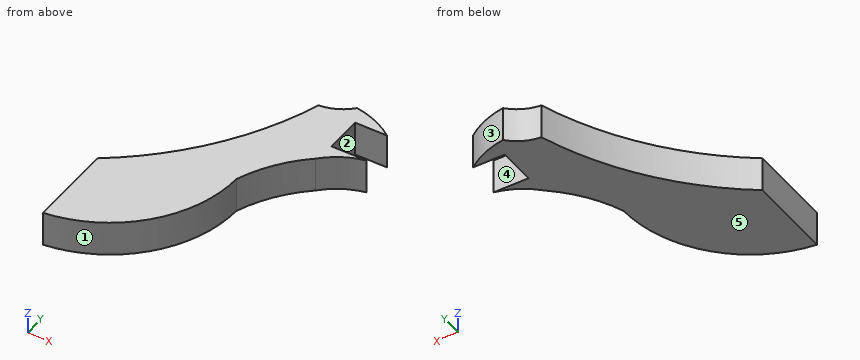
from build123d import *

# Parameters (mm, degrees)
BOSS_EXTRUDE1_DEPTH = 1.524


with BuildPart() as part:
    # Sketch1 → Boss-Extrude1 (new body)
    with BuildSketch(Plane.XY):
        with BuildLine():
            Line((110.824360774, -1.524), (109.29292347, -1.524))
            Line((109.29292347, -1.524), (109.29292347, 0.099254425))
            Line((109.29292347, 0.099254425), (110.685720546, 0.099254425))
            ThreePointArc((110.685720546, 0.099254425), (109.844126395, 0.589914025), (108.904790048, 0.848128638))
            ThreePointArc((108.904790048, 0.848128638), (108.321557599, 0.411980775), (107.618800979, 0.220883469))
            ThreePointArc((107.618800979, 0.220883469), (105.564728066, -3.682348009), (102.379001913, -6.732852948))
            Line((102.379001913, -6.732852948), (102.379001913, -10.469177864))
            ThreePointArc((102.379001913, -10.469177864), (105.901664911, -8.680555585), (107.348345234, -5.004220414))
            ThreePointArc((107.348345234, -5.004220414), (108.094332128, -3.601037602), (109.178159994, -2.438826088))
            ThreePointArc((109.178159994, -2.438826088), (109.930755444, -1.854541621), (110.824360774, -1.524))
        make_face()
    extrude(amount=BOSS_EXTRUDE1_DEPTH)


solid = part.part
For this review, take the finished solid that the model builds, in its own axes (mm). Face numbers are marked on the shaded views. A direction names the side the tool comes from. Round coordinates to 2 decimals unless told otherwise and drop trailing zeros. Loops run counter-clockwise (first coordinate to the right, second up) from the corner with the lowest first, then second, coordinate; pieces in that order, holes last. Notation, with made-up numbers: (89.25, 46) - (121.25, 46) arc R24 ccw to (121.25, 79) - close; hole circle Ø4 at (73.5, 68.5). An arc over 180 degrees is marked (long way). One line per question, with ' | ' between items.
Q1. For line 1 along X through (y, z) = (-7.25, 1.1); line 2 along Y through (x, z) = (103, 0.7); line 3 along Y through (x, z) = (106.25, 0.6), list the stretches that pass through material, from the lowest coordinate up. Write a range as [from, to].
Taken from the geometry:
line 1: x = [102.38, 106.85] | line 2: y = [-10.37, -6.28] | line 3: y = [-8.26, -2.68]
Q2. The part is to be moulded in two halves that separate along Y. For the marked faces 1, 2 and 3, say which applies: released by +Y, released by -Y, zero draft, split by the parting line, or undercut.
Taken from the geometry:
face 1: released by -Y | face 2: undercut | face 3: released by +Y
Q3. Take a section at C-C (y = -8.5). Give the boundary of the cut face in (x, z), and give its area (3 significant figures).
Taken from the geometry:
outline: (102.38, 0) - (106.06, 0) - (106.06, 1.52) - (102.38, 1.52) - close | area: 5.61 mm²
Q4. Take a section at A-A (z = 0.4). Give the boundary of the cut face in (x, y), and give its area (3 significant figures).
Taken from the geometry:
outline: (102.38, -10.47) arc R5.56 ccw to (107.35, -5) arc R6.09 cw to (109.18, -2.44) arc R3.13 cw to (110.82, -1.52) - (109.29, -1.52) - (109.29, 0.1) - (110.69, 0.1) arc R3.76 ccw to (108.9, 0.85) arc R1.95 cw to (107.62, 0.22) arc R13.73 cw to (102.38, -6.73) - close | area: 32.9 mm²
Q5. Take a section at B-B (x = 104.75). Give the boundary of the cut face in (y, z).
Taken from the geometry:
outline: (-9.65, 0) - (-4.66, 0) - (-4.66, 1.52) - (-9.65, 1.52) - close
Q6. Tool access review of the marked faces 4 and 5: name each direction out of +Z, -Z, +X, -X, +Y, -Y from which nothing blocks a thin tool from reaching the whole face with its end or side.
Taken from the geometry:
face 4: +Z, -Z, +X | face 5: -Z, +X, -X, +Y, -Y
Q7. For pin 1 (3 mm diameter, centred on x = 103.5, y = -0.5, fed in from +Z), flat-tipped, find the tip position at first contact; note if it passes through.
Taken from the geometry:
pin 1: passes through
